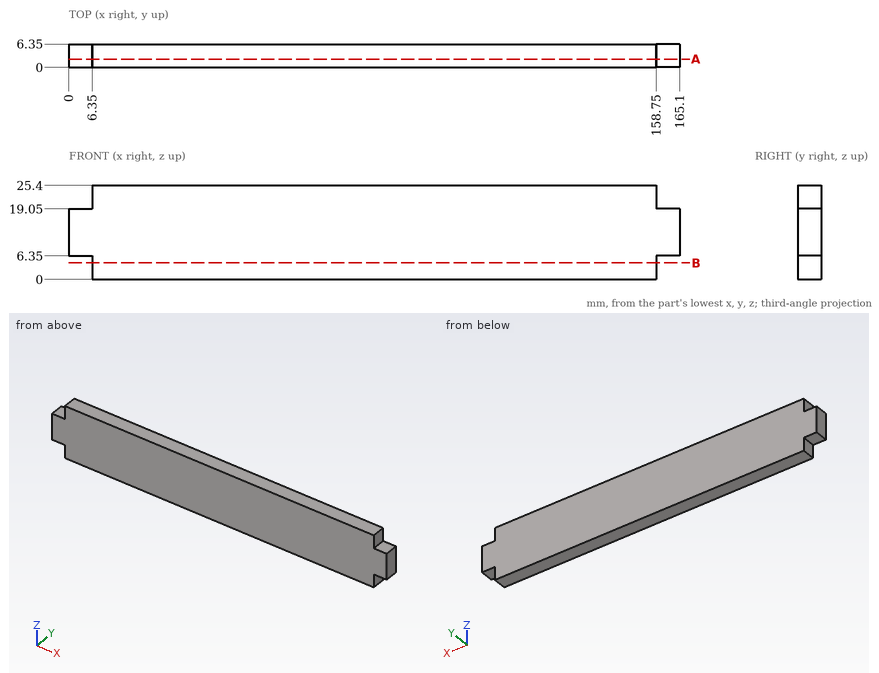
Here's the drawing with two shaded views (mm, measured from the low corner). I have some questions. Coordinates: 2 decimals unless noted, no trailing zeros. Write each loop counter-clockwise with the first axis right and the second up, starting at its lowest first coordinate (ties: lowest second). Pieces come first, ordered by that corner, then holes. Notation, with made-up numbers: M -35,-32.5 L -14,-32.5 A26 cw -14,6.5 Z; hole C 55.25,-39 d5. An arc over 180 degrees is marked long. Answer as CSV lines item,"result".
Item 1: Imagine slicing it at A-A on y = 2.25. List the corners of the cut face in (x, z) for me, plus the area to 3 significant figures.
Geometry results:
outline,"M 0,6.35 L 6.35,6.35 L 6.35,0 L 158.75,0 L 158.75,6.35 L 165.1,6.35 L 165.1,19.05 L 158.75,19.05 L 158.75,25.4 L 6.35,25.4 L 6.35,19.05 L 0,19.05 Z"
area,"4,030 mm2"
Item 2: Please list where this line runs through material, in increasing order: line 1 along X through (y, z) = (5, 2.75).
Geometry results:
line 1,"x = 6.35 to 158.75"
Item 3: Imagine slicing it at B-B on z = 4.5. List the corners of the cut face in (x, y) for me.
Geometry results:
outline,"M 6.35,0 L 158.75,0 L 158.75,6.35 L 6.35,6.35 Z"
Item 4: I'm going to push flat-ended pins straight in: P1, Ø3, axis at y = 2, z = 4, coming from the +X side; P2, Ø2, axis at x = 122, y = 5, coming from the -Z side; P3, Ø1.9, axis at x = 163.5, y = 3, coming from the +Z side. Where does each tip first touch, or does it pass through?
Geometry results:
P1,"stops at x = 158.75"
P2,"stops at z = 0"
P3,"stops at z = 19.05"
